Can you work these out from the model? Positions are in its coordinate system, mm. A direction names the side the tool comes from. Round coordinates to 2 decimals unless told otherwise and drop trailing zeros. Order: outer loops, then holes, each group sorted by start corner. A loop starts at its lowest first (then second) coordinate and runs counter-clockwise, first axis right, second up. Notation, with made-up numbers: (-27, -31) - (8, -31) arc R21 ccw to (8, -4) - close; hole circle Ø11 at (83.5, 13). An arc over 180 degrees is marked (long way). Write item = value, one per line.
from build123d import *

# Parameters (mm, degrees)
CROQUIS1_W                   = 44.5
CROQUIS1_H                   = 44.5
CROQUIS1_W_2                 = 39.5
CROQUIS1_H_2                 = 39.5
SALIENTE_EXTRUIR1_DEPTH      = 40
SALIENTE_EXTRUIR1_DEPTH_BACK = 40
CORTAR_EXTRUIR1_DEPTH        = 44.5
SALIENTE_EXTRUIR2_DEPTH      = 1.25
SALIENTE_EXTRUIR2_DEPTH_BACK = 1.25
CROQUIS4_R                   = 5
CORTAR_EXTRUIR2_DEPTH        = 2.5
CROQUIS7_R                   = 12
CORTAR_EXTRUIR5_DEPTH        = 2.5
CROQUIS8_R                   = 2.25
CORTAR_EXTRUIR6_DEPTH        = 2.5


with BuildPart() as part:
    # Croquis1 → Saliente-Extruir1 (new body, two sides)
    with BuildSketch(Plane.XY) as saliente_extruir1_sk:
        Rectangle(CROQUIS1_W, CROQUIS1_H)
        Rectangle(CROQUIS1_W_2, CROQUIS1_H_2, mode=Mode.SUBTRACT)
    extrude(amount=SALIENTE_EXTRUIR1_DEPTH)
    extrude(saliente_extruir1_sk.sketch, amount=-SALIENTE_EXTRUIR1_DEPTH_BACK)

    # Croquis2 → Cortar-Extruir1 (cut)
    with BuildSketch(Plane(origin=(22.25, 0, 0), x_dir=(0, 0, -1), z_dir=(1, 0, 0))):
        Polygon((-9.620253165, 10.25), (9.620253165, 10.25), (40, -19.75), (40, 22.25), (-40, 22.25), (-40, -19.75), align=None)
    extrude(amount=-CORTAR_EXTRUIR1_DEPTH, mode=Mode.SUBTRACT)

    # Croquis3 → Saliente-Extruir2 (add, two sides)
    with BuildSketch(Plane.XY) as saliente_extruir2_sk:
        Polygon((19.75, -19.75), (19.75, 10.25), (7.75, 22.25), (-7.75, 22.25), (-19.75, 10.25), (-19.75, -19.75), align=None)
    extrude(amount=SALIENTE_EXTRUIR2_DEPTH)
    extrude(saliente_extruir2_sk.sketch, amount=-SALIENTE_EXTRUIR2_DEPTH_BACK)

    # Croquis4 → Cortar-Extruir2 (cut)
    with BuildSketch(Plane.XZ.offset(22.25)):
        with Locations((0, -20)):
            Circle(CROQUIS4_R)
        with Locations((0, 20)):
            Circle(CROQUIS4_R)
    extrude(amount=-CORTAR_EXTRUIR2_DEPTH, mode=Mode.SUBTRACT)

    # Croquis7 → Cortar-Extruir5 (cut)
    with BuildSketch(Plane.XY.offset(1.25)):
        with Locations((0, 9.75)):
            Circle(CROQUIS7_R)
    extrude(amount=-CORTAR_EXTRUIR5_DEPTH, mode=Mode.SUBTRACT)

    # Croquis8 → Cortar-Extruir6 (cut)
    with BuildSketch(Plane.XY.offset(1.25)):
        with Locations((-11.37991652, 21.35)):
            Circle(CROQUIS8_R)
        with Locations((11.37991652, 21.35)):
            Circle(CROQUIS8_R)
        with Locations((-16.25, 9.75)):
            Circle(CROQUIS8_R)
        with Locations((16.25, 9.75)):
            Circle(CROQUIS8_R)
        with Locations((-11.37991652, -1.85)):
            Circle(CROQUIS8_R)
        with Locations((11.37991652, -1.85)):
            Circle(CROQUIS8_R)
    extrude(amount=-CORTAR_EXTRUIR6_DEPTH, mode=Mode.SUBTRACT)


solid = part.part
(1) Will these pins go through, and if not, where does the flat tip stop? P1, Ø5, axis at x = 16.25, y = 9.75, coming from the -Z side; P2, Ø1.2, axis at x = -20.5, z = 2, coming from the +Y side; P3, Ø11.5, axis at x = 5, z = 17, coming from the +Y side.
Computed:
P1 = -1.25
P2 = 10.25
P3 = -19.75
(2) If I drill on line 1 (Z direction, x = 0, y = -21); line 2 (Y direction, x = 0, z = -0.7); line 3 (X direction, y = 0, z = 4.5), over which ranges is the centre line in solid material (lowest first)? Write a range as from..to.
Computed:
line_1 = -40..-25, -15..15, 25..40
line_2 = -22.25..-2.25, 21.75..22.25
line_3 = -22.25..-19.75, 19.75..22.25
(3) If we section it at C-C (y = 13): Write out the boundary of the cut face in (x, z), plus the area to 3 significant figures.
Computed:
outline = (-17, -1.25) - (-11.55, -1.25) - (-11.55, 1.25) - (-17, 1.25) - close; (11.55, -1.25) - (17, -1.25) - (17, 1.25) - (11.55, 1.25) - close
area = 27.2 mm^2
(4) Thinking about a two-plate mould opening in Y: for faces 4 (the face through (22.25, -10, 1)), 5 (the face through (-8.844, 17.86, 0.018)), 6 (the face through (0, -22.25, 1)), 7 (the face through (21.02, -4.54, -24.6)), which applies, +Y half, -Y half, draft (parallel to the pull), parting line (faces both ways), or undercut?
Computed:
face_4 = draft
face_5 = undercut
face_6 = -Y half
face_7 = +Y half
(5) If we section it at B-B (z = -20): Write out the boundary of the cut face in (x, y).
Computed:
outline = (-22.25, -22.25) - (-5, -22.25) - (-5, -19.75) - (-19.75, -19.75) - (-19.75, 0) - (-22.25, 0) - close; (5, -22.25) - (22.25, -22.25) - (22.25, 0) - (19.75, 0) - (19.75, -19.75) - (5, -19.75) - close
(6) If we section it at D-D (x = 0): Write out the boundary of the cut face in (y, z).
Computed:
outline = (-22.25, -40) - (-19.75, -40) - (-19.75, -25) - (-22.25, -25) - close; (-22.25, -15) - (-19.75, -15) - (-19.75, -1.25) - (-2.25, -1.25) - (-2.25, 1.25) - (-19.75, 1.25) - (-19.75, 15) - (-22.25, 15) - close; (-22.25, 25) - (-19.75, 25) - (-19.75, 40) - (-22.25, 40) - close; (21.75, -1.25) - (22.25, -1.25) - (22.25, 1.25) - (21.75, 1.25) - close
(7) If we section it at A-A (x = 16.25): Write out the boundary of the cut face in (y, z), plus the area to 4 significant figures.
Computed:
outline = (-22.25, -40) - (-19.75, -40) - (-19.75, -1.25) - (7.5, -1.25) - (7.5, 1.25) - (-19.75, 1.25) - (-19.75, 40) - (-22.25, 40) - close; (12, -1.25) - (13.75, -1.25) - (13.75, 1.25) - (12, 1.25) - close
area = 272.5 mm^2
(8) On a 3-axis mill with a long thin cutter (end or side, diameter ignored), from which of +Z, -Z, +X, -X, +Y, -Y can I reach the whole of each face in a straight line? I mean faces 1 (the face through (-15.04, 11.647, 0.018)), 2 (the face through (-19.75, -8, -16)), 3 (the face through (-19.75, -8, 17)). Say none if no direction works.
Computed:
face_1 = +Z, -Z
face_2 = -Z, +Y
face_3 = +Z, +Y
